The model under review builds one solid part; all positions refer to its coordinate system, in mm. Coordinates: 2 decimals unless noted, no trailing zeros. Order: outer loops, then holes, each group sorted by start corner. A loop starts at its lowest first (then second) coordinate and runs counter-clockwise, first axis right, second up. Notation, with made-up numbers: M -34,6.5 L -2,6.5 A33 cw -2,36.5 Z; hole C -37,3 d11. An arc over 180 degrees is marked long. Answer as CSV lines item,"result". Start each with the question number.
Q1. Wall thickness on L1, parallel to Y at x = -17, z = 1.75; L2, parallel to Z at x = 146, y = -88: over which ranges is each line inside the solid? List them lowest first. Write a range as [from, to].
Q2. Consider section A-A on x = -229.5. Write out the cut boundary in (y, z), and give its area (3 significant figures).
Q3. For P1, Ø0.6, axis at x = 331, z = 1, coming from the +Y side; P2, Ø1.6, axis at x = -50.5, z = 0.5, coming from the -Y side; P3, Ø1.5, axis at x = -279.5, y = -62.5, coming from the -Z side, all flat-tipped, find the tip position at first contact; note any pin that passes through.
Q4. The part is to be moulded in two halves that separate along X. For faces 1 (the face through (-375, -1, 9)), 2 (the face through (375, -1, 9)), 3 (the face through (-5, -100, 10)), 4 (the face through (26, -89, 2)), say which applies: +X half, -X half, draft (parallel to the pull), parting line (faces both ways), or undercut.
from build123d import *

# Parameters (mm, degrees)
SKETCH1_W           = 750
SKETCH1_H           = 200
BOSS_EXTRUDE1_DEPTH = 18
SKETCH2_W           = 2
SKETCH2_H           = 18
CUT_EXTRUDE3_DEPTH  = 757.851372464
SKETCH3_W           = 18
SKETCH3_H           = 328.758100902
SKETCH3_H_2         = 372.829020194
SKETCH3_H_3         = 369.502918338
SKETCH3_H_4         = 384.006512989
SKETCH3_H_5         = 390.144460662
CUT_EXTRUDE4_DEPTH  = 2


with BuildPart() as part:
    # Sketch1 → Boss-Extrude1 (new body)
    with BuildSketch(Plane.XY):
        Rectangle(SKETCH1_W, SKETCH1_H)
    extrude(amount=BOSS_EXTRUDE1_DEPTH)

    # Sketch2 → Cut-Extrude3 (cut, through all)
    with BuildSketch(Plane.ZY.offset(375)):
        with Locations((1, -91)):
            Rectangle(SKETCH2_W, SKETCH2_H)
        with Locations((1, 91)):
            Rectangle(SKETCH2_W, SKETCH2_H)
    extrude(amount=-CUT_EXTRUDE3_DEPTH, mode=Mode.SUBTRACT)

    # Sketch3 → Cut-Extrude4 (cut)
    with BuildSketch(Plane(origin=(0, 0, 0), x_dir=(-1, 0, 0), z_dir=(0, 0, -1))):
        with Locations((276, 27.416436842)):
            Rectangle(SKETCH3_W, SKETCH3_H)
        with Locations((138, 25.675959121)):
            Rectangle(SKETCH3_W, SKETCH3_H_2)
        with Locations((0, 35.637467242)):
            Rectangle(SKETCH3_W, SKETCH3_H_3)
        with Locations((-138, 42.889264568)):
            Rectangle(SKETCH3_W, SKETCH3_H_4)
        with Locations((-276, 58.109616722)):
            Rectangle(SKETCH3_W, SKETCH3_H_5)
    extrude(amount=-CUT_EXTRUDE4_DEPTH, mode=Mode.SUBTRACT)


solid = part.part
Evaluation:
1,L1,"y = [-82, 82]"
1,L2,"z = [2, 18]"
2,outline,"M -100,2 L -82,2 L -82,0 L 82,0 L 82,2 L 100,2 L 100,18 L -100,18 Z"
2,area,"3,530 mm²"
3,P1,"stops at y = 82"
3,P2,"stops at y = -82"
3,P3,"stops at z = 2"
4,face 1,"-X half"
4,face 2,"+X half"
4,face 3,"draft"
4,face 4,"undercut"
